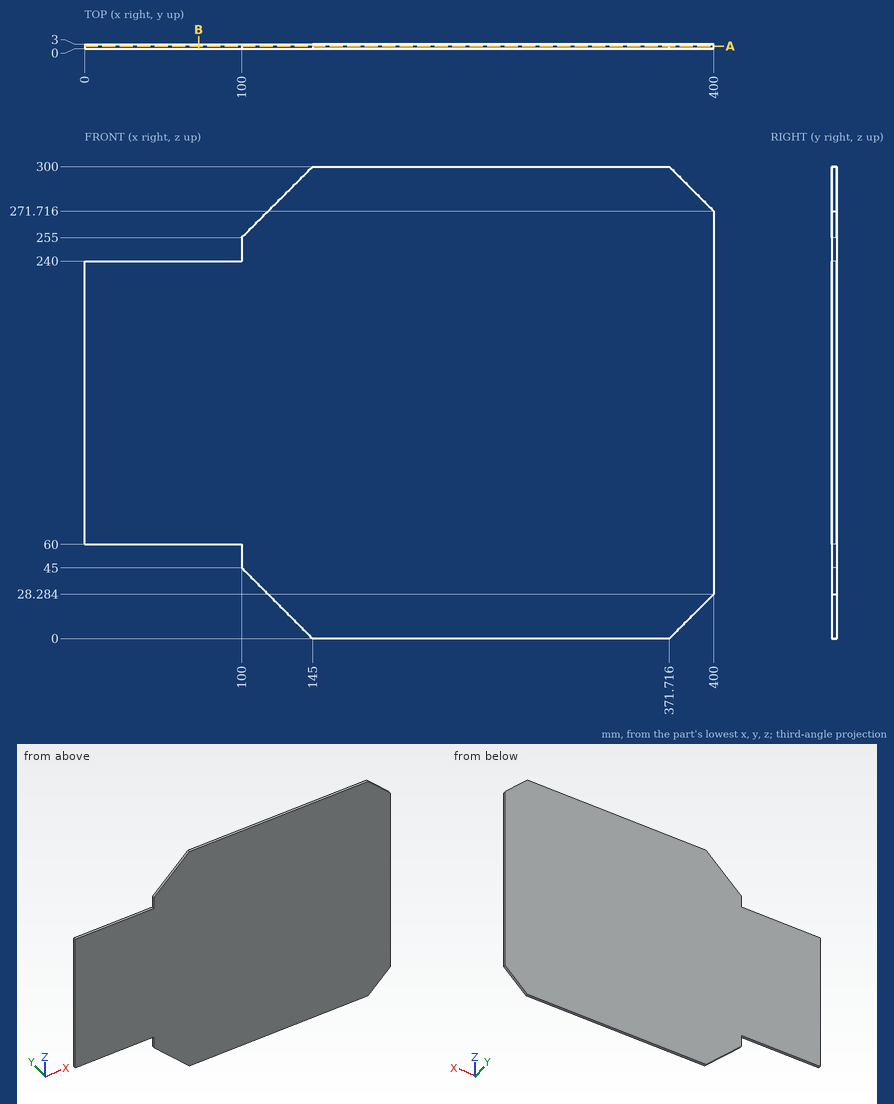
For this review, use the dimensioned drawing (mm, ordinates from the lowest corner) and the shaded views. Round coordinates to 2 decimals unless told otherwise and drop trailing zeros. Loops run counter-clockwise (first coordinate to the right, second up) from the corner with the lowest first, then second, coordinate; pieces in that order, holes last. Notation, with made-up numbers: M 58.5,36 L 105.5,36 A21 ccw 105.5,56 Z; hole C 82.25,88 d2. An arc over 180 degrees is marked long. Answer as CSV lines item,"result".
1. We need section A-A (y = 1.6). Give the boundary of the cut face in (x, z).
Outcome:
outline,"M 0,60 L 100,60 L 100,45 L 145,0 L 371.72,0 L 400,28.28 L 400,271.72 L 371.72,300 L 145,300 L 100,255 L 100,240 L 0,240 Z"
2. Insertion check: pin 1 Ø1.5 at (x, y) = (67, 1.5) entering from -Z; pin 2 Ø1.5 at (y, z) = (1.5, 55.5) entering from -X. Each pin has a flat end and moves straight along its axis. Give the tip position at first contact, or say it passes through.
Outcome:
pin 1,"stops at z = 60"
pin 2,"stops at x = 100"
3. To check wall thickness, follow L1, parallel to Z at x = 42, y = 0.4; L2, parallel to X at y = 2.8, z = 50; L3, parallel to X at y = 2.2, z = 44.5. State the ranges of each line that lie inside material, in increasing order. Write a range as [from, to].
Outcome:
L1,"z = [60, 240]"
L2,"x = [100, 400]"
L3,"x = [100.5, 400]"
4. We need section B-B (x = 72.5). Give the boundary of the cut face in (y, z).
Outcome:
outline,"M 0,60 L 3,60 L 3,240 L 0,240 Z"
